```python
from build123d import *

# Parameters (mm, degrees)
BOSS_EXTRUDE1_DEPTH = 4
FILLET1_R           = 7.62
FILLET2_R           = 7.62


with BuildPart() as part:
    # Sketch1 → Boss-Extrude1 (new body)
    with BuildSketch(Plane(origin=(0, 0, 0), x_dir=(0, 0, -1), z_dir=(1, 0, 0))):
        with BuildLine():
            Line((-0.858815867, 31.104520152), (27.081184133, 31.104520152))
            ThreePointArc((27.081184133, 31.104520152), (38.755701446, 36.548436981), (42.089654289, 48.99091838))
            Line((42.089654289, 48.99091838), (27.309926766, 132.81091838))
            ThreePointArc((27.309926766, 132.81091838), (22.097539782, 141.839037466), (12.30145661, 145.404520152))
            Line((12.30145661, 145.404520152), (-11.714075954, 145.404520152))
            ThreePointArc((-11.714075954, 145.404520152), (-24.518671733, 140.524264284), (-30.82684486, 128.359498679))
            add(Edge.make_bspline(
                [(-30.82684486, 128.359498679), (-1.209368429, 86.647497598), (-30.82684486, 48.99091838)],
                knots=[0, 0, 0, 1, 1, 1], degree=2))
            ThreePointArc((-30.82684486, 48.99091838), (-18.308787237, 35.916095552), (-0.858815867, 31.104520152))
        make_face()
    extrude(amount=BOSS_EXTRUDE1_DEPTH)

    # Fillet1
    fillet1_edges = [part.edges().sort_by_distance(p)[0] for p in [
        (2, 128.359498679, 30.82684486),
    ]]
    fillet(fillet1_edges, radius=FILLET1_R)

    # Fillet2
    fillet2_edges = [part.edges().sort_by_distance(p)[0] for p in [
        (2, 48.99091838, 30.82684486),
    ]]
    fillet(fillet2_edges, radius=FILLET2_R)


solid = part.part
```
For this review, take the finished solid that the model builds, in its own axes (mm). Round coordinates to 2 decimals unless told otherwise and drop trailing zeros. Loops run counter-clockwise (first coordinate to the right, second up) from the corner with the lowest first, then second, coordinate; pieces in that order, holes last.
(1) Wall thickness on line 1 along Z through (x, y) = (3.5, 139); line 2 along Z through (x, y) = (0.9, 137.5); line 3 along Y through (x, z) = (2.5, 24.5): over which ranges is each line inside the solid? List them lowest first.
Returned:
line 1: z = -24.72 to 26.05
line 2: z = -25.66 to 27.26
line 3: y = 40.65 to 58.21, 118.28 to 140.54
(2) We need section A-A (z = -34.5). Give the boundary of the cut face in (x, y), plus the area to 3 significant figures.
Returned:
outline: (0, 33.03) - (4, 33.03) - (4, 92.03) - (0, 92.03) - close
area: 236 mm2
(3) We need section B-B (y = 39.5). Give the boundary of the cut face in (x, z).
Returned:
outline: (0, -40.7) - (4, -40.7) - (4, 23.25) - (0, 23.25) - close
(4) Clearance check with flat-ended pins moving along their axes: P1, Ø2, axis at x = 1.5, y = 107.5, coming from the -Z side; P2, Ø1, axis at x = 0.5, y = 63.5, coming from the +Z side. State where each tip first meets the part, or that it passes through.
Returned:
P1: stops at z = -31.95
P2: stops at z = 21.93
